Part model, mm, in its own coordinate system. Face numbers are marked on the shaded views. A direction names the side the tool comes from. Coordinates: 2 decimals unless noted, no trailing zeros. Write each loop counter-clockwise with the first axis right and the second up, starting at its lowest first coordinate (ties: lowest second). Pieces come first, ordered by that corner, then holes. Notation, with made-up numbers: (23, 88) - (49, 88) arc R13 cw to (49, 94) - close; hole circle Ø1 at (-16, 82). An arc over 180 degrees is marked (long way). Use one line per item in the form item = value. Start each with the question number.
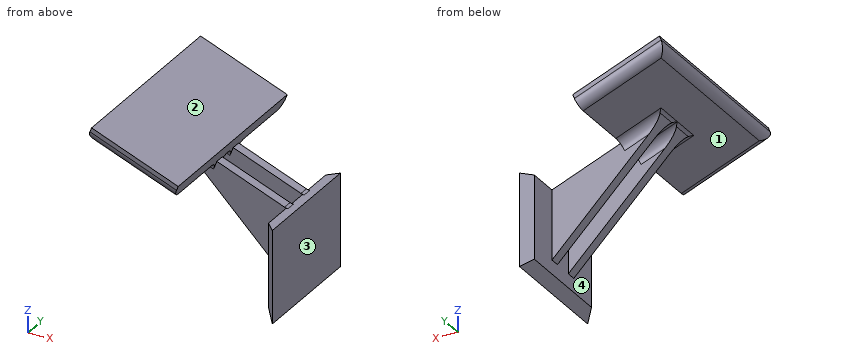
from build123d import *

# Parameters (mm, degrees)
SKETCH1_W           = 25
SKETCH1_H           = 20
BOSS_EXTRUDE1_DEPTH = 2
BOSS_EXTRUDE2_DEPTH = 4
CUT_EXTRUDE1_DEPTH  = 2
SKETCH5_W           = 20
SKETCH5_H           = 40
BOSS_EXTRUDE5_DEPTH = 3
FILLET3_R           = 2
CHAMFER1_SIZE       = 2
FILLET4_R           = 2


with BuildPart() as part:
    # Sketch1 → Boss-Extrude1 (new body)
    with BuildSketch(Plane.YZ):
        Rectangle(SKETCH1_W, SKETCH1_H)
    extrude(amount=BOSS_EXTRUDE1_DEPTH)

    # Sketch2 → Boss-Extrude2 (add, symmetric)
    with BuildSketch(Plane(origin=(0, 0, 0), x_dir=(-1, 0, 0), z_dir=(0, 1, 0))):
        Polygon((0, -5), (24.285410332, 19.285410332), (0, 10), align=None)
    extrude(amount=BOSS_EXTRUDE2_DEPTH, both=True)

    # Sketch2<2> → Cut-Extrude1 (cut, symmetric)
    with BuildSketch(Plane(origin=(0, 0, 0), x_dir=(-1, 0, 0), z_dir=(0, 1, 0))):
        Polygon((0, -5), (24.285410332, 19.285410332), (0, 10), align=None)
    extrude(amount=CUT_EXTRUDE1_DEPTH, both=True, mode=Mode.SUBTRACT)

    # Sketch5 → Boss-Extrude5 (add)
    with BuildSketch(Plane(origin=(3.335798817, 0, 8.724573298), x_dir=(0.9340542435228668, 0, -0.3571311665997872), z_dir=(0.3571311665997872, 0, 0.9340542435228668))):
        with Locations((-29.571311666, 0)):
            Rectangle(SKETCH5_W, SKETCH5_H)
    extrude(amount=BOSS_EXTRUDE5_DEPTH)

    # Fillet3
    fillet3_edges = [part.edges().sort_by_distance(p)[0] for p in [
        (-19.615139114, -4, 17.499754499),
        (-24.285410332, 3, 19.285410332),
        (-19.615139114, 4, 17.499754499),
        (-24.285410332, -3, 19.285410332),
        (-19.615139114, -2, 17.499754499),
        (-19.615139114, 2, 17.499754499),
        (-33.625952767, 0, 22.856721998),
        (-24.285410332, -20, 19.285410332),
        (-24.285410332, 20, 19.285410332),
    ]]
    fillet(fillet3_edges, radius=FILLET3_R - 0.0001)  # a hair under: the kernel refuses the full size

    # Chamfer1
    chamfer1_edges = [part.edges().sort_by_distance(p)[0] for p in [
        (0, -12.5, 0),
        (0, 0, -10),
        (0, 12.5, 0),
    ]]
    chamfer(chamfer1_edges, length=CHAMFER1_SIZE - 0.0001)  # a hair under: the kernel refuses the full size

    # Fillet4
    fillet4_edges = [part.edges().sort_by_distance(p)[0] for p in [
        (0, 3, 10),
        (0, -3, 10),
    ]]
    fillet(fillet4_edges, radius=FILLET4_R)


solid = part.part
Q1. Which spindle directions (+Z, -Z, +X, -X, +Y, -Y) get a long thin tool onto all of the face, cutting with end or side? Do the marked faces 1 and 2. Say none if no direction does.
Q2. Slice it at C-C (x = -1). List the corners of the cut face in (y, z).
Q3. Drill centre lines: probe 1 along Y at (x, z) = (-16, 13); probe 2 along X at (y, z) = (-5.5, -4.5); probe 3 along Z at (x, y) = (-18, 10). Where is each one in solid material? Low to high.
Q4. Mould opens along Y. For the marked faces 3 and 4 say: released by +Y, released by -Y, zero draft, split by the parting line, or undercut.
Q5. Slice it at D-D (z = 13). List the corners of the cut face in (x, y), plus the area to 3 significant figures.
Q6. Pin check, flat tips, straight feed: P1, Ø16.5, axis at x = -13, z = 3, coming from the -Y side; P2, Ø1, axis at y = -0.5, z = 3, coming from the -X side; P3, Ø16.5, axis at x = -8, z = 6, coming from the -Y side. Stop position of each tip, or through.
Solution:
q1.face_1 = -Z, -X
q1.face_2 = +Z, +X, +Y, -Y
q2.outline = (-4, -4) - (-2, -4) - (-2, 10.38) - (-4, 10.38) - close; (2, -4) - (4, -4) - (4, 10.38) - (2, 10.38) - close
q3.probe_1 = -4 to -2, 2 to 4
q3.probe_2 = 0 to 2
q3.probe_3 = 16.88 to 20.09
q4.face_3 = zero draft
q4.face_4 = undercut
q5.outline = (-18, -4) - (-7.85, -4) - (-7.85, -2) - (-18, -2) - close; (-18, 2) - (-7.85, 2) - (-7.85, 4) - (-18, 4) - close
q5.area = 40.6 mm2
q6.P1 = -4
q6.P2 = 0
q6.P3 = -10.75
